Build history of the part. All positions in model axes, mm. A direction names the side the tool comes from. Round coordinates to 2 decimals unless told otherwise and drop trailing zeros. Loops run counter-clockwise (first coordinate to the right, second up) from the corner with the lowest first, then second, coordinate; pieces in that order, holes last.
from build123d import *

# Parameters (mm, degrees)
TOP_W                                     = 12
TOP_H                                     = 10
PRECISION_MICRODRIVES_MODEL_212_109_DEPTH = 24
TOP_RING_2_R                              = 2
TOP_RING_DEPTH                            = 0.7
HOLE_WIZARD_M1_1_D                        = 1.1
HOLE_WIZARD_M1_1_DEPTH                    = 10
HOLE_WIZARD_M1_1_TIP                      = 0.337040433
HOLE_WIZARD_M1_2_D                        = 1.1
HOLE_WIZARD_M1_2_DEPTH                    = 10
HOLE_WIZARD_M1_2_TIP                      = 0.337040433
D_SHAFT_DEPTH                             = 8
VERRUNDUNG1_R                             = 3
SKIZZE12_R                                = 2.5
BOTTOM_DEPTH                              = 1.2
SKIZZE13_R                                = 0.5
BOLT_DEPTH                                = 6
SKIZZE14_W                                = 0.12
SKIZZE14_H                                = 1.5
FLAPS_DEPTH                               = 2.5
FLAP1_CUT_REACH                           = 11.56
SKIZZE15_R                                = 0.4
FLAP2_CUT_REACH                           = 11.56
SKIZZE16_R                                = 0.4
SKIZZE21_W                                = 12
SKIZZE21_H                                = 9
AUFSATZ_LINEAR_AUSTRAGEN2_DEPTH           = 10
SKIZZE22_W                                = 6
SKIZZE22_H                                = 15
SCHNITT_LINEAR_AUSTRAGEN3_DEPTH           = 0.01
SKIZZE23_W                                = 15
SKIZZE23_H                                = 4
SCHNITT_LINEAR_AUSTRAGEN4_DEPTH           = 0.01
SKIZZE24_W                                = 6
SKIZZE24_H                                = 15
SCHNITT_LINEAR_AUSTRAGEN5_DEPTH           = 0.01
SKIZZE25_W                                = 15
SKIZZE25_H                                = 4
SCHNITT_LINEAR_AUSTRAGEN6_DEPTH           = 0.01
VERRUNDUNG2_R                             = 0.5


with BuildPart() as part:
    # top → Precision Microdrives Model 212-109 (new body)
    with BuildSketch(Plane.XY):
        Rectangle(TOP_W, TOP_H)
    extrude(amount=-PRECISION_MICRODRIVES_MODEL_212_109_DEPTH)

    # top ring 2 → top-ring (add)
    with BuildSketch(Plane.XY):
        Circle(TOP_RING_2_R)
    extrude(amount=TOP_RING_DEPTH)

    # Hole Wizard M1-1
    with Locations(Plane.XY):
        with Locations((-4.5, 0)):
            Hole(HOLE_WIZARD_M1_1_D / 2, depth=HOLE_WIZARD_M1_1_DEPTH)
            with Locations((0, 0, -(HOLE_WIZARD_M1_1_DEPTH + HOLE_WIZARD_M1_1_TIP / 2))):  # 117° drill point
                Cone(0, HOLE_WIZARD_M1_1_D / 2, HOLE_WIZARD_M1_1_TIP, mode=Mode.SUBTRACT)

    # Hole Wizard M1-2
    with Locations(Plane.XY):
        with Locations((4.5, 0)):
            Hole(HOLE_WIZARD_M1_2_D / 2, depth=HOLE_WIZARD_M1_2_DEPTH)
            with Locations((0, 0, -(HOLE_WIZARD_M1_2_DEPTH + HOLE_WIZARD_M1_2_TIP / 2))):  # 117° drill point
                Cone(0, HOLE_WIZARD_M1_2_D / 2, HOLE_WIZARD_M1_2_TIP, mode=Mode.SUBTRACT)

    # Skizze11 → D-Shaft (add)
    with BuildSketch(Plane.XY):
        with BuildLine():
            Line((-1.071214264, 1.05), (1.071214264, 1.05))
            ThreePointArc((1.071214264, 1.05), (0, -1.5), (-1.071214264, 1.05))
        make_face()
    extrude(amount=D_SHAFT_DEPTH)

    # Verrundung1
    verrundung1_edges = [part.edges().sort_by_distance(p)[0] for p in [
        (-6, 5, -12),
        (6, 5, -12),
        (6, -5, -12),
        (-6, -5, -12),
    ]]
    fillet(verrundung1_edges, radius=VERRUNDUNG1_R)

    # Skizze12 → bottom (add)
    with BuildSketch(Plane(origin=(0, 0, -24), x_dir=(-1, 0, 0), z_dir=(0, 0, -1))):
        Circle(SKIZZE12_R)
    extrude(amount=BOTTOM_DEPTH)

    # Skizze13 → bolt (add)
    with BuildSketch(Plane(origin=(0, 0, -24), x_dir=(-1, 0, 0), z_dir=(0, 0, -1))):
        Circle(SKIZZE13_R)
    extrude(amount=BOLT_DEPTH)

    # Skizze14 → flaps (add)
    with BuildSketch(Plane(origin=(0, 0, -24), x_dir=(-1, 0, 0), z_dir=(0, 0, -1))):
        with Locations((-3.5, 0)):
            Rectangle(SKIZZE14_W, SKIZZE14_H)
        with Locations((3.5, 0)):
            Rectangle(SKIZZE14_W, SKIZZE14_H)
    extrude(amount=FLAPS_DEPTH)

    # Skizze15 → flap1-cut (cut, up to next)
    with BuildSketch(Plane.ZY.offset(3.56), mode=Mode.PRIVATE) as flap1_cut_sk1:
        with Locations((-25.7, 0)):
            Circle(SKIZZE15_R)
    flap1_cut_tool1 = extrude(flap1_cut_sk1.sketch, amount=-FLAP1_CUT_REACH, mode=Mode.PRIVATE) & part.part
    add(flap1_cut_tool1.solids().sort_by_distance((-3.56, 0, -25.7))[0], mode=Mode.SUBTRACT)

    # Skizze16 → flap2-cut (cut, up to next)
    with BuildSketch(Plane(origin=(3.56, 0, 0), x_dir=(0, 0, -1), z_dir=(1, 0, 0)), mode=Mode.PRIVATE) as flap2_cut_sk1:
        with Locations((25.7, 0)):
            Circle(SKIZZE16_R)
    flap2_cut_tool1 = extrude(flap2_cut_sk1.sketch, amount=-FLAP2_CUT_REACH, mode=Mode.PRIVATE) & part.part
    add(flap2_cut_tool1.solids().sort_by_distance((3.56, 0, -25.7))[0], mode=Mode.SUBTRACT)

    # Skizze21 → Aufsatz-Linear austragen2 (add)
    with BuildSketch(Plane(origin=(0, 5, 0), x_dir=(1, 0, 0), z_dir=(0, 1, 0))):
        with Locations((0, 4.5)):
            Rectangle(SKIZZE21_W, SKIZZE21_H)
    extrude(amount=-AUFSATZ_LINEAR_AUSTRAGEN2_DEPTH)

    # Skizze22 → Schnitt-Linear austragen3 (cut)
    with BuildSketch(Plane.XZ.offset(5)):
        with Locations((0, -16.5)):
            Rectangle(SKIZZE22_W, SKIZZE22_H)
    extrude(amount=-SCHNITT_LINEAR_AUSTRAGEN3_DEPTH, mode=Mode.SUBTRACT)

    # Skizze23 → Schnitt-Linear austragen4 (cut)
    with BuildSketch(Plane(origin=(6, 0, 0), x_dir=(0, 0, -1), z_dir=(1, 0, 0))):
        with Locations((16.5, 0)):
            Rectangle(SKIZZE23_W, SKIZZE23_H)
    extrude(amount=-SCHNITT_LINEAR_AUSTRAGEN4_DEPTH, mode=Mode.SUBTRACT)

    # Skizze24 → Schnitt-Linear austragen5 (cut)
    with BuildSketch(Plane(origin=(0, 5, 0), x_dir=(1, 0, 0), z_dir=(0, 1, 0))):
        with Locations((0, 16.5)):
            Rectangle(SKIZZE24_W, SKIZZE24_H)
    extrude(amount=-SCHNITT_LINEAR_AUSTRAGEN5_DEPTH, mode=Mode.SUBTRACT)

    # Skizze25 → Schnitt-Linear austragen6 (cut)
    with BuildSketch(Plane.ZY.offset(6)):
        with Locations((-16.5, 0)):
            Rectangle(SKIZZE25_W, SKIZZE25_H)
    extrude(amount=-SCHNITT_LINEAR_AUSTRAGEN6_DEPTH, mode=Mode.SUBTRACT)

    # Verrundung2
    verrundung2_edges = [part.edges().sort_by_distance(p)[0] for p in [
        (-6, 5, -4.5),
        (6, -5, -4.5),
        (-6, -5, -4.5),
        (6, 5, -4.5),
    ]]
    fillet(verrundung2_edges, radius=VERRUNDUNG2_R)


solid = part.part
(1) Pull direction Y, two halves, no side cores. Call faces 4 (the face through (-0.434, -1.952, 0.345)), 5 (the face through (0, 0, -30)), 6 (the face through (-4.595, 0.004, -10.279)): +Y half, -Y half, draft (parallel to the pull), parting line (faces both ways), or undercut.
Responses:
face 4: parting line
face 5: draft
face 6: undercut
(2) Which spindle directions (+Z, -Z, +X, -X, +Y, -Y) get a long thin tool onto all of the face, cutting with end or side? Do faces 1 (the face through (0.54, -2.44, -24.59)), 2 (the face through (3.99, -0.21, -9.51)), 3 (the face through (0, -1.5, 4.3)). Say none if no direction does.
Responses:
face 1: -Z
face 2: none
face 3: +Z
(3) Slice it at A-A on z = -25.7. List the corners of the cut face in (x, y).
Responses:
outline: (-3.56, -0.75) - (-3.44, -0.75) - (-3.44, -0.4) - (-3.56, -0.4) - close; (-3.56, 0.4) - (-3.44, 0.4) - (-3.44, 0.75) - (-3.56, 0.75) - close; circle Ø1 at (0, 0); (3.44, -0.75) - (3.56, -0.75) - (3.56, -0.4) - (3.44, -0.4) - close; (3.44, 0.4) - (3.56, 0.4) - (3.56, 0.75) - (3.44, 0.75) - close
(4) Slice it at D-D on z = 2. List the corners of the cut face in (x, y), plus the area to 3 significant figures.
Responses:
outline: (-1.07, 1.05) arc R1.5 ccw (long way) to (1.07, 1.05) - close
area: 6.40 mm2
(5) Pin check, flat tips, straight feed: P1, Ø5, axis at x = 2.5, z = 3.5, coming from the -Y side; P2, Ø1.2, axis at x = -4.5, y = 0, coming from the -Z side; P3, Ø1, axis at x = -3.5, z = -13, coming from the +Y side; P4, Ø1.6, axis at y = 0, z = -25, coming from the +X side. Stop position of each tip, or through.
Responses:
P1: stops at y = -1.5
P2: stops at z = -24
P3: stops at y = 5
P4: stops at x = 3.56
(6) Probe line 1 (Y direction, x = -3.5, z = -25.7); line 2 (X direction, y = 0, z = -9.15); line 3 (Z direction, x = -1, y = 3). List the from-to ranges inside material, lowest first.
Responses:
line 1: y = -0.75 to -0.4, 0.4 to 0.75
line 2: x = -5.99 to -5.05, -3.95 to 3.95, 5.05 to 5.99
line 3: z = -24 to 0
(7) Slice it at C-C on y = 3.25. List the corners of the cut face in (x, z).
Responses:
outline: (-6, -9) - (-5.73, -9) - (-5.73, -24) - (5.73, -24) - (5.73, -9) - (6, -9) - (6, 0) - (-6, 0) - close
